Geometry check sheet. Reference: the model listing, model coordinates, mm. Coordinates: 2 decimals unless noted, no trailing zeros. Loops run counter-clockwise (first coordinate to the right, second up) from the corner with the lowest first, then second, coordinate; pieces in that order, holes last.
from build123d import *

# Parameters (mm, degrees)
F1_DEPTH = 1
F2_R     = 1


with BuildPart() as f1:
    # F0 (on Top) → F1 (new body)
    with BuildSketch(Plane.XY):
        with BuildLine():
            ThreePointArc((-2.5, 0), (-1.767766953, 1.767766953), (0, 2.5))
            ThreePointArc((0, 2.5), (-1.2472191289, 2.9365280801), (-1.9499920861, 4.0555555556))
            ThreePointArc((-1.9499920861, 4.0555555556), (-3.1819805153, 3.1819805153), (-4.0555555556, 1.9499920861))
            ThreePointArc((-4.0555555556, 1.9499920861), (-2.9365280801, 1.2472191289), (-2.5, 0))
        make_face()
        with BuildLine():
            Line((-3.45, 0), (-2.5, 0))
            ThreePointArc((-2.5, 0), (-2.9365280801, 1.2472191289), (-4.0555555556, 1.9499920861))
            ThreePointArc((-4.0555555556, 1.9499920861), (-4.2408539714, 1.5050440503), (-4.3775, 1.0428296841))
            ThreePointArc((-4.3775, 1.0428296841), (-3.715422088, 0.6978090713), (-3.45, 0))
        make_face()
        with BuildLine():
            ThreePointArc((-4.0555555556, -1.9499920861), (-2.9365280801, -1.2472191289), (-2.5, 0))
            Line((-2.5, 0), (-3.45, 0))
            ThreePointArc((-3.45, 0), (-3.715422088, -0.6978090713), (-4.3775, -1.0428296841))
            ThreePointArc((-4.3775, -1.0428296841), (-4.2408539714, -1.5050440503), (-4.0555555556, -1.9499920861))
        make_face()
        with BuildLine():
            ThreePointArc((-1.9499920861, -4.0555555556), (-1.2472191276, -2.936528079), (3.3e-09, -2.5))
            ThreePointArc((3.3e-09, -2.5), (-1.7677669518, -1.7677669542), (-2.5, 0))
            ThreePointArc((-2.5, 0), (-2.9365280801, -1.2472191289), (-4.0555555556, -1.9499920861))
            ThreePointArc((-4.0555555556, -1.9499920861), (-3.1819805153, -3.1819805153), (-1.9499920861, -4.0555555556))
        make_face()
        with BuildLine():
            ThreePointArc((4.0555555556, -1.9499920861), (2.9365280801, -1.2472191289), (2.5, 0))
            ThreePointArc((2.5, 0), (1.7677669542, -1.7677669518), (3.3e-09, -2.5))
            ThreePointArc((3.3e-09, -2.5), (1.2472191302, -2.9365280811), (1.9499920861, -4.0555555556))
            ThreePointArc((1.9499920861, -4.0555555556), (3.1819805153, -3.1819805153), (4.0555555556, -1.9499920861))
        make_face()
        with BuildLine():
            Line((3.45, 0), (2.5, 0))
            ThreePointArc((2.5, 0), (2.9365280801, -1.2472191289), (4.0555555556, -1.9499920861))
            ThreePointArc((4.0555555556, -1.9499920861), (4.2408539714, -1.5050440503), (4.3775, -1.0428296841))
            ThreePointArc((4.3775, -1.0428296841), (3.715422088, -0.6978090713), (3.45, 0))
        make_face()
        with BuildLine():
            ThreePointArc((4.0555555556, 1.9499920861), (2.9365280801, 1.2472191289), (2.5, 0))
            Line((2.5, 0), (3.45, 0))
            ThreePointArc((3.45, 0), (3.715422088, 0.6978090713), (4.3775, 1.0428296841))
            ThreePointArc((4.3775, 1.0428296841), (4.2408539714, 1.5050440503), (4.0555555556, 1.9499920861))
        make_face()
        with BuildLine():
            ThreePointArc((0, 2.5), (1.767766953, 1.767766953), (2.5, 0))
            ThreePointArc((2.5, 0), (2.9365280801, 1.2472191289), (4.0555555556, 1.9499920861))
            ThreePointArc((4.0555555556, 1.9499920861), (3.1819805153, 3.1819805153), (1.9499920861, 4.0555555556))
            ThreePointArc((1.9499920861, 4.0555555556), (1.2472191289, 2.9365280801), (0, 2.5))
        make_face()
        with BuildLine():
            Line((0, 3.45), (0, 2.5))
            ThreePointArc((0, 2.5), (1.2472191289, 2.9365280801), (1.9499920861, 4.0555555556))
            ThreePointArc((1.9499920861, 4.0555555556), (1.5050440503, 4.2408539714), (1.0428296841, 4.3775))
            ThreePointArc((1.0428296841, 4.3775), (0.6978090713, 3.715422088), (0, 3.45))
        make_face()
        with BuildLine():
            ThreePointArc((-1.9499920861, 4.0555555556), (-1.2472191289, 2.9365280801), (0, 2.5))
            Line((0, 2.5), (0, 3.45))
            ThreePointArc((0, 3.45), (-0.6978090713, 3.715422088), (-1.0428296841, 4.3775))
            ThreePointArc((-1.0428296841, 4.3775), (-1.5050440503, 4.2408539714), (-1.9499920861, 4.0555555556))
        make_face()
        with BuildLine():
            ThreePointArc((0, 6.5), (-1.5634719199, 5.7472191289), (-1.9499920861, 4.0555555556))
            ThreePointArc((-1.9499920861, 4.0555555556), (-1.5050440503, 4.2408539714), (-1.0428296841, 4.3775))
            ThreePointArc((-1.0428296841, 4.3775), (-0.784577912, 5.1978090713), (0, 5.55))
            Line((0, 5.55), (0, 6.5))
        make_face()
        with BuildLine():
            ThreePointArc((1.0428296841, 4.3775), (1.5050440503, 4.2408539714), (1.9499920861, 4.0555555556))
            ThreePointArc((1.9499920861, 4.0555555556), (1.9874587005, 4.2763755069), (2, 4.5))
            ThreePointArc((2, 4.5), (1.4142135624, 5.9142135624), (0, 6.5))
            Line((0, 6.5), (0, 5.55))
            ThreePointArc((0, 5.55), (0.7424621202, 5.2424621202), (1.05, 4.5))
            ThreePointArc((1.05, 4.5), (1.0482058882, 4.4386451644), (1.0428296841, 4.3775))
        make_face()
        with BuildLine():
            ThreePointArc((6.5, 0), (5.7472191289, 1.5634719199), (4.0555555556, 1.9499920861))
            ThreePointArc((4.0555555556, 1.9499920861), (4.2408539714, 1.5050440503), (4.3775, 1.0428296841))
            ThreePointArc((4.3775, 1.0428296841), (5.1978090713, 0.784577912), (5.55, 0))
            Line((5.55, 0), (6.5, 0))
        make_face()
        with BuildLine():
            ThreePointArc((4.3775, -1.0428296841), (4.2408539714, -1.5050440503), (4.0555555556, -1.9499920861))
            ThreePointArc((4.0555555556, -1.9499920861), (5.7472191289, -1.5634719199), (6.5, 0))
            Line((6.5, 0), (5.55, 0))
            ThreePointArc((5.55, 0), (5.1978090713, -0.784577912), (4.3775, -1.0428296841))
        make_face()
        with BuildLine():
            ThreePointArc((1.9499920861, -4.0555555556), (1.2472191302, -2.9365280811), (3.3e-09, -2.5))
            Line((0, -2.5), (0, -3.45))
            ThreePointArc((0, -3.45), (0.6978090713, -3.715422088), (1.0428296841, -4.3775))
            ThreePointArc((1.0428296841, -4.3775), (1.5050440503, -4.2408539714), (1.9499920861, -4.0555555556))
        make_face()
        with BuildLine():
            Line((0, -3.45), (0, -2.5))
            ThreePointArc((3.3e-09, -2.5), (-1.2472191276, -2.936528079), (-1.9499920861, -4.0555555556))
            ThreePointArc((-1.9499920861, -4.0555555556), (-1.5050440503, -4.2408539714), (-1.0428296841, -4.3775))
            ThreePointArc((-1.0428296841, -4.3775), (-0.6978090713, -3.715422088), (0, -3.45))
        make_face()
        with BuildLine():
            ThreePointArc((-1.0428296841, -4.3775), (-1.5050440503, -4.2408539714), (-1.9499920861, -4.0555555556))
            ThreePointArc((-1.9499920861, -4.0555555556), (-1.5634719204, -5.7472191284), (-1.3e-09, -6.5))
            Line((0, -6.5), (0, -5.55))
            ThreePointArc((0, -5.55), (-0.784577912, -5.1978090713), (-1.0428296841, -4.3775))
        make_face()
        with BuildLine():
            ThreePointArc((2, -4.5), (1.9874587005, -4.2763755069), (1.9499920861, -4.0555555556))
            ThreePointArc((1.9499920861, -4.0555555556), (1.5050440503, -4.2408539714), (1.0428296841, -4.3775))
            ThreePointArc((1.0428296841, -4.3775), (1.0482058882, -4.4386451644), (1.05, -4.5))
            ThreePointArc((1.05, -4.5), (0.7424621202, -5.2424621202), (0, -5.55))
            Line((0, -5.55), (0, -6.5))
            ThreePointArc((-1.3e-09, -6.5), (1.4142135619, -5.9142135628), (2, -4.5))
        make_face()
        with BuildLine():
            ThreePointArc((-6.5, 2.4e-09), (-5.7472191299, -1.5634719192), (-4.0555555556, -1.9499920861))
            ThreePointArc((-4.0555555556, -1.9499920861), (-4.2408539714, -1.5050440503), (-4.3775, -1.0428296841))
            ThreePointArc((-4.3775, -1.0428296841), (-5.1978090713, -0.784577912), (-5.55, 0))
            Line((-5.55, 0), (-6.5, 0))
        make_face()
        with BuildLine():
            ThreePointArc((-4.3775, 1.0428296841), (-4.2408539714, 1.5050440503), (-4.0555555556, 1.9499920861))
            ThreePointArc((-4.0555555556, 1.9499920861), (-5.747219128, 1.5634719207), (-6.5, 2.4e-09))
            Line((-6.5, 0), (-5.55, 0))
            ThreePointArc((-5.55, 0), (-5.1978090713, 0.784577912), (-4.3775, 1.0428296841))
        make_face()
    extrude(amount=F1_DEPTH)

    # F2
    f2_edges = [f1.edges().sort_by_distance(p)[0] for p in [
        (-4.055556, 1.949992, 0.5),
        (-1.949992, 4.055556, 0.5),
        (1.949992, 4.055556, 0.5),
        (4.055556, 1.949992, 0.5),
        (4.055556, -1.949992, 0.5),
        (1.949992, -4.055556, 0.5),
        (-1.949992, -4.055556, 0.5),
        (-4.055556, -1.949992, 0.5),
    ]]
    fillet(f2_edges, radius=F2_R)


solid = f1.part
1) Section check D-D on y = 3. Record the cut outline in (x, z), and give its area (3 significant figures).
Data:
outline: (-3.35, 0) - (3.35, 0) - (3.35, 1) - (-3.35, 1) - close
area: 6.71 mm2
2) Section check A-A on x = 1.5. Record the cut outline in (y, z), and give its area (3 significant figures).
Data:
outline: (-5.82, 0) - (-2, 0) - (-2, 1) - (-5.82, 1) - close; (2, 0) - (5.82, 0) - (5.82, 1) - (2, 1) - close
area: 7.65 mm2
3) Section check C-C on z = 0.25. Count the separate pieces of the cut face and the enclosed holes in it, and give its area (3 significant figures).
Data:
separate pieces: 1
enclosed holes: 5
area: 58.1 mm2
4) Section check B-B on y = -5. Record the cut outline in (x, z).
Data:
outline: (-1.94, 0) - (-0.92, 0) - (-0.92, 1) - (-1.94, 1) - close; (0.92, 0) - (1.94, 0) - (1.94, 1) - (0.92, 1) - close
5) Mould release check, pull along Z, two halves, no side actions. Record for faces 1 (the flat face through (0, -3, 0)), 2 (the flat face through (0, -3, 1)), 3 (the cylindrical face through (3.191, 3.173, 0.493)): +Z half, -Z half, draft (parallel to the pull), parting line (faces both ways), or undercut.
Data:
face 1: -Z half
face 2: +Z half
face 3: draft
6) Material ranges on probe 1 along X at (y, z) = (0.5, 0.9); probe 2 along Y at (x, z) = (-1.5, 0.65), recorded low to high.
Data:
probe 1: x = -6.44 to -5.42, -3.58 to -2.45, 2.45 to 3.58, 5.42 to 6.44
probe 2: y = -5.82 to -2, 2 to 5.82
